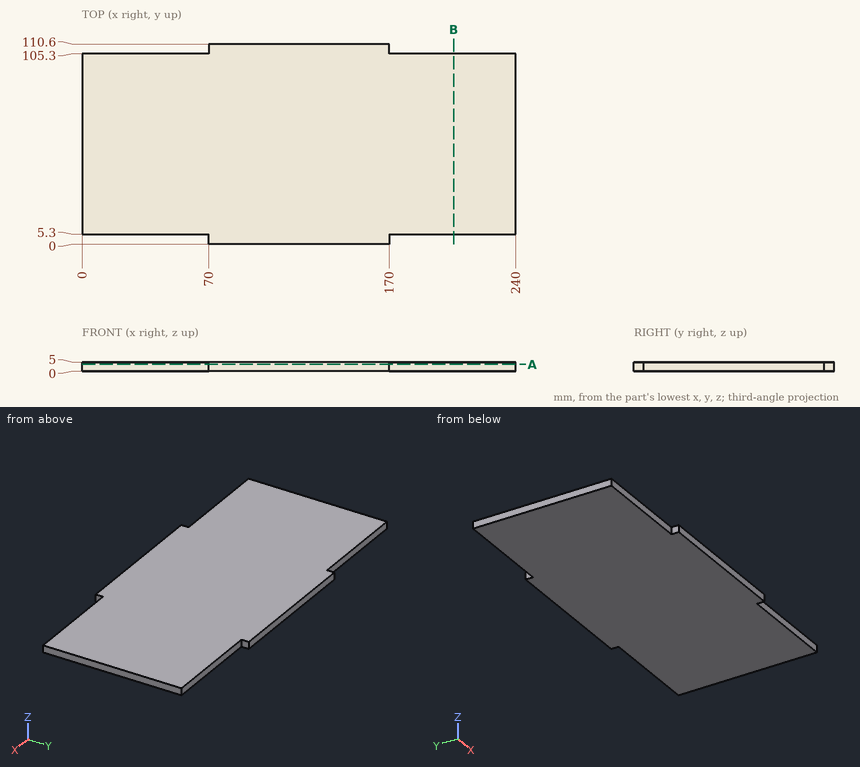
Design review of the part shown in the three views and the two pictorial views. Dimensions are in mm from the part's minimum x, y and z. Round coordinates to 2 decimals unless told otherwise and drop trailing zeros. Write each loop counter-clockwise with the first axis right and the second up, starting at its lowest first coordinate (ties: lowest second). Pieces come first, ordered by that corner, then holes.
Item 1: We need section B-B on x = 205.5. Write out the cut boundary in (y, z).
Item 2: We need section A-A on z = 3.75. Write out the cut boundary in (x, y).
Item 3: For probe 1 along Y at (x, z) = (36, 2.5); probe 2 along X at (y, z) = (5, 0.6), list the stretches that pass through material, from the lowest coordinate up.
Item 4: Clearance check with flat-ended pins moving along their axes: pin 1 Ø2.5 at (x, z) = (30.5, 3) entering from +Y; pin 2 Ø2.5 at (y, z) = (107, 2.5) entering from +X; pin 3 Ø2.5 at (x, z) = (31, 2) entering from -Y. State where each tip first meets the part, or that it passes through.
Returned:
1. outline: (5.3, 0) - (105.3, 0) - (105.3, 5) - (5.3, 5) - close
2. outline: (0, 5.3) - (70, 5.3) - (70, 0) - (170, 0) - (170, 5.3) - (240, 5.3) - (240, 105.3) - (170, 105.3) - (170, 110.6) - (70, 110.6) - (70, 105.3) - (0, 105.3) - close
3. probe 1: y = 5.3 to 105.3
3. probe 2: x = 70 to 170
4. pin 1: stops at y = 105.3
4. pin 2: stops at x = 170
4. pin 3: stops at y = 5.3
